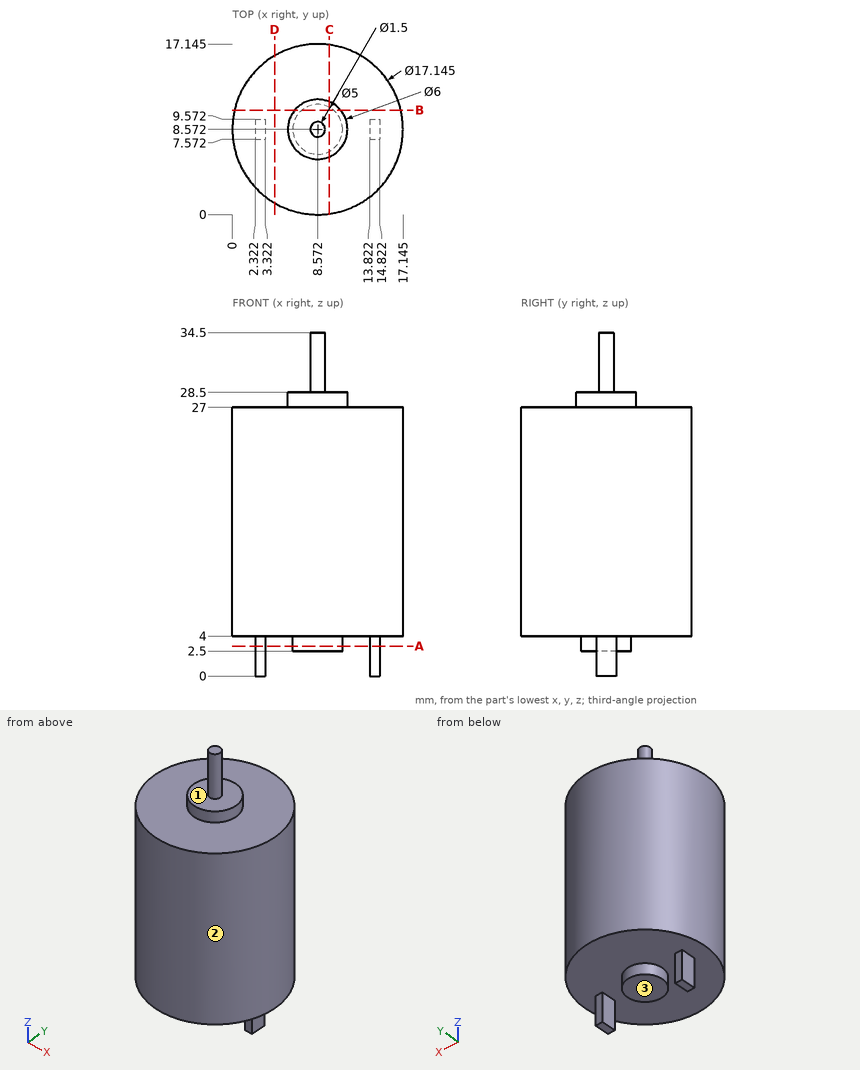
Study the drawing (mm; zero at the part's minimum x, y, z) and answer. Coordinates: 2 decimals unless noted, no trailing zeros. Write each loop counter-clockwise with the first axis right and the second up, starting at its lowest first coordinate (ties: lowest second). Pieces come first, ordered by that corner, then holes. Notation, with made-up numbers: (-30.75, 19.5) - (-7.75, 19.5) arc R12 ccw to (-7.75, 38.5) - close; hole circle Ø5 at (16, 46.25). An arc over 180 degrees is marked (long way). Answer as a JSON object with one key per item and string values. Group by question number.
1. A cutting plane is placed at B-B (y = 10.5). Determine the outline of the cut face in (x, z) (1 decimal), plus the area to 3 significant figures.
2. Consider L1, parallel to Z at x = 12, y = 5.75; L2, parallel to Y at x = 3.25, z = 2; L3, parallel to Z at x = 10.25, y = 7.5. Determine where each line is inside the solid, lowest interval first. Write a range as [from, to].
3. Each of these flat-tipped pins is pushed along its axis until it touches: P1, Ø10, axis at x = 7.5, z = 17.5, coming from the +Y side (1 decimal); P2, Ø0.6, axis at y = 8.5, z = 2.5, coming from the +X side; P3, Ø5, axis at x = 12, z = 27.5, coming from the -Y side; P4, Ø0.8, axis at x = 3, z = 1, coming from the +Y side. Where does it stop, or does it pass through?
4. A cutting plane is placed at C-C (x = 9.75). Determine the outline of the cut face in (y, z).
5. A cutting plane is placed at D-D (x = 4.25). Determine the outline of the cut face in (y, z) (1 decimal).
6. The mould has two halves that part along X. Classify the marked faces 1, 2 and 3: +X half, -X half, draft (parallel to the pull), parting line (faces both ways), or undercut.
7. A cutting plane is placed at A-A (z = 3). Determine the outline of the cut face in (x, y).
Worked out:
{
 "1": {"outline": "(0.2, 4) - (7, 4) - (7, 2.5) - (10.2, 2.5) - (10.2, 4) - (16.9, 4) - (16.9, 27) - (10.9, 27) - (10.9, 28.5) - (6.3, 28.5) - (6.3, 27) - (0.2, 27) - close", "area": "396 mm²"},
 "2": {"L1": "z = [4, 27]", "L2": "y = [7.57, 9.57]", "L3": "z = [2.5, 28.5]"},
 "3": {"P1": "stops at y = 17.1", "P2": "stops at x = 14.82", "P3": "stops at y = 0.06", "P4": "stops at y = 9.57"},
 "4": {"outline": "(0.08, 4) - (6.37, 4) - (6.37, 2.5) - (10.78, 2.5) - (10.78, 4) - (17.06, 4) - (17.06, 27) - (11.33, 27) - (11.33, 28.5) - (5.81, 28.5) - (5.81, 27) - (0.08, 27) - close"},
 "5": {"outline": "(1.2, 4) - (16, 4) - (16, 27) - (1.2, 27) - close"},
 "6": {"face 1": "draft", "face 2": "parting line", "face 3": "undercut"},
 "7": {"outline": "(2.32, 7.57) - (3.32, 7.57) - (3.32, 9.57) - (2.32, 9.57) - close; circle Ø5 at (8.57, 8.57); (13.82, 7.57) - (14.82, 7.57) - (14.82, 9.57) - (13.82, 9.57) - close"}
}
